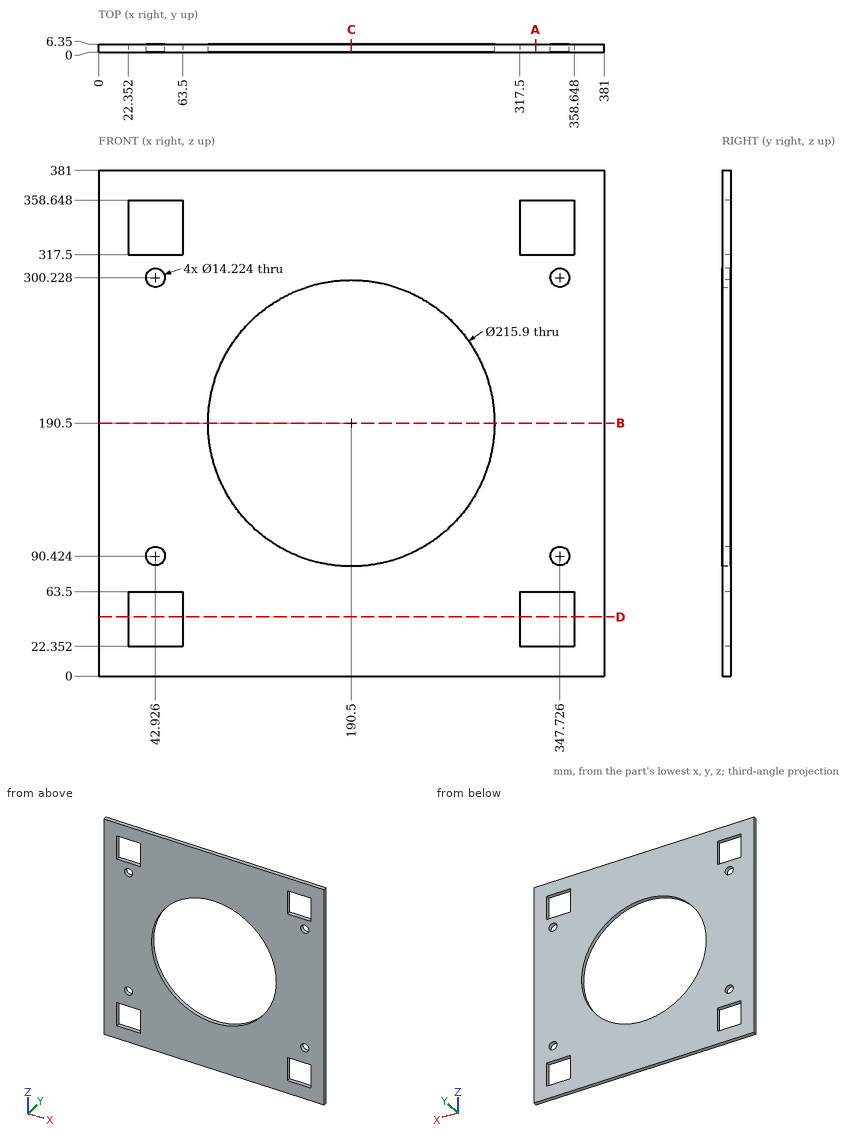
Design review of the part shown in the three views and the two pictorial views. Dimensions are in mm from the part's minimum x, y and z. Round coordinates to 2 decimals unless told otherwise and drop trailing zeros. Order: outer loops, then holes, each group sorted by start corner. A loop starts at its lowest first (then second) coordinate and runs counter-clockwise, first axis right, second up.
(1) Wall thickness on L1, parallel to Z at x = 27, y = 5.25; L2, parallel to X at y = 1.75, z = 190.5; L3, parallel to X at y = 5.75, z = 164: over which ranges is each line inside the solid? List them lowest first.
Working result:
L1: z = 0 to 22.35, 63.5 to 317.5, 358.65 to 381
L2: x = 0 to 82.55, 298.45 to 381
L3: x = 0 to 85.85, 295.15 to 381
(2) Take a section at B-B, the plane z = 190.5. State the section outline as (x, y) points.
Working result:
outline: (0, 0) - (82.55, 0) - (82.55, 6.35) - (0, 6.35) - close; (298.45, 0) - (381, 0) - (381, 6.35) - (298.45, 6.35) - close
(3) Take a section at C-C, the plane x = 190.5. State the section outline as (y, z) points, plus the area to 3 significant figures.
Working result:
outline: (0, 0) - (6.35, 0) - (6.35, 82.55) - (0, 82.55) - close; (0, 298.45) - (6.35, 298.45) - (6.35, 381) - (0, 381) - close
area: 1,050 mm2
(4) Take a section at A-A, the plane x = 329.5. State the section outline as (y, z) points.
Working result:
outline: (0, 0) - (6.35, 0) - (6.35, 22.35) - (0, 22.35) - close; (0, 63.5) - (6.35, 63.5) - (6.35, 317.5) - (0, 317.5) - close; (0, 358.65) - (6.35, 358.65) - (6.35, 381) - (0, 381) - close
(5) Take a section at D-D, the plane z = 44.5. State the section outline as (x, y) points, plus the area to 3 significant figures.
Working result:
outline: (0, 0) - (22.35, 0) - (22.35, 6.35) - (0, 6.35) - close; (63.5, 0) - (317.5, 0) - (317.5, 6.35) - (63.5, 6.35) - close; (358.65, 0) - (381, 0) - (381, 6.35) - (358.65, 6.35) - close
area: 1,900 mm2
